from build123d import *

# Parameters (mm, degrees)
F0_W      = 400
F0_H      = 400
F1_DEPTH  = 100
F1_TAPER  = 15
F2_W      = 146.4101615138
F2_H      = 146.4101615138
F3_DEPTH  = 100
F3_TAPER  = 10
F4_R      = 20
F5_R      = 20
F6_DEPTH  = 50
F7_W      = 100
F7_H      = 200
F7_R      = 20
F8_DEPTH  = 10
F9_W      = 100
F9_H      = 10
F10_DEPTH = 75
F11_R     = 5


with BuildPart() as f1:
    # F0 (on Top) → F1 (new body)
    with BuildSketch(Plane.XY):
        with Locations((200, 200)):
            Rectangle(F0_W, F0_H)
    extrude(amount=F1_DEPTH, taper=F1_TAPER)

    # F2 (on face) → F3 (join)
    with BuildSketch(Plane.XY.offset(100)):
        with Locations((200, 200)):
            Rectangle(F2_W, F2_H)
    extrude(amount=F3_DEPTH, taper=F3_TAPER)

    # F4
    f4_edges = [f1.edges().sort_by_distance(p)[0] for p in [
        (13.39746, 13.39746, 50),
        (386.60254, 13.39746, 50),
        (13.39746, 386.60254, 50),
        (386.60254, 386.60254, 50),
        (200, 373.205081, 100),
        (26.794919, 200, 100),
        (200, 26.794919, 100),
        (373.205081, 200, 100),
        (273.205081, 200, 100),
        (200, 126.794919, 100),
        (264.388732, 135.611268, 150),
        (126.794919, 200, 100),
        (135.611268, 135.611268, 150),
        (200, 273.205081, 100),
        (264.388731, 264.388731, 150.000003),
        (135.611268, 264.388732, 150),
    ]]
    fillet(f4_edges, radius=F4_R)

    # F5 (on face) → F6 (join)
    with BuildSketch(Plane.XY.offset(200)):
        with Locations((200, 200)):
            Circle(F5_R)
    extrude(amount=F6_DEPTH)

    # F7 (on face) → F8 (join)
    with BuildSketch(Plane.XY.offset(250)):
        with Locations((200, 200)):
            Rectangle(F7_W, F7_H)
        with Locations((200, 200)):
            Circle(F7_R, mode=Mode.SUBTRACT)
        with Locations((200, 200)):
            Circle(F7_R)
    extrude(amount=F8_DEPTH)

    # F9 (on face) → F10 (join)
    with BuildSketch(Plane.XY.offset(260)):
        with Locations((200, 295)):
            Rectangle(F9_W, F9_H)
    extrude(amount=F10_DEPTH)

    # F11
    f11_edges = [f1.edges().sort_by_distance(p)[0] for p in [
        (200, 290, 260),
        (200, 300, 250),
    ]]
    fillet(f11_edges, radius=F11_R)


solid = f1.part
Read the model definition and answer for the solid it produces. Units are mm, in the model's axes. A direction names the side the tool comes from. Coordinates: 2 decimals unless noted, no trailing zeros. Loops run counter-clockwise (first coordinate to the right, second up) from the corner with the lowest first, then second, coordinate; pieces in that order, holes last.
Q1. The part is cut by section C-C on y = 93. Write down the section's boundary in (x, z), and give its area (3 significant figures).
Q2. Which of the six approach directions +Z, -Z, +X, -X, +Y, -Y give full straight-line access (tool end or side, diameter ignored) to faces 1 (the face through (250, 222, 258)), 2 (the face through (199.292, 263.035, 157.679)), 3 (the face through (150, 222, 258))?
Q3. Consider probe 1 along Z at (x, y) = (267, 322.5); probe 2 along Y at (x, z) = (179, 294.5); probe 3 along Y at (x, z) = (202, 156.5). Determine where each line is inside the solid, lowest interval first.
Q4. The part is cut by section B-B on y = 200. Write down the section's boundary in (x, z), and give its area (3 significant figures).
Q5. Each of these flat-tipped pins is pushed along its axis until it touches: pin 1 Ø5 at (x, z) = (184, 256.5) entering from -Y; pin 2 Ø1 at (x, y) = (278.5, 242) entering from +Z; pin 3 Ø5 at (x, z) = (223.5, 142.5) entering from -Y; pin 4 Ø10 at (x, y) = (146.5, 297) entering from +Z. Where does it stop, or does it pass through?
Q6. The part is cut by section A-A on x = 200. Write down the section's boundary in (y, z), and give its area (3 significant figures).
Q7. The mould has two halves that part along Z. Classify faces 4 (the face through (257.274, 256.969, 158.693)), 5 (the face through (197.79, 370.179, 95.755)), 6 (the face through (199, 290, 300)): +Z half, -Z half, draft (parallel to the pull), parting line (faces both ways), or undercut.
Results below:
1. outline: (0, 0) - (400, 0) - (377.18, 85.18) arc R20 ccw to (357.86, 100) - (42.14, 100) arc R20 ccw to (22.82, 85.18) - close
1. area: 37,200 mm2
2. face 1: +Z, +X, +Y, -Y
2. face 2: +X, -X, +Y
2. face 3: +Z, -X, +Y, -Y
3. probe 1: z = 0 to 100
3. probe 2: y = 290 to 300
3. probe 3: y = 136.76 to 263.24
4. outline: (0, 0) - (400, 0) - (377.18, 85.18) arc R20 ccw to (357.86, 100) - (289.99, 100) arc R20 cw to (270.29, 116.53) - (255.57, 200) - (220, 200) - (220, 250) - (250, 250) - (250, 260) - (150, 260) - (150, 250) - (180, 250) - (180, 200) - (144.43, 200) - (129.71, 116.53) arc R20 cw to (110.01, 100) - (42.14, 100) arc R20 ccw to (22.82, 85.18) - close
4. area: 53,200 mm2
5. pin 1: stops at y = 100
5. pin 2: stops at z = 103.99
5. pin 3: stops at y = 133.85
5. pin 4: stops at z = 335
6. outline: (0, 0) - (400, 0) - (377.18, 85.18) arc R20 ccw to (357.86, 100) - (289.99, 100) arc R20 cw to (270.29, 116.53) - (255.57, 200) - (220, 200) - (220, 250) - (295, 250) arc R5 ccw to (300, 255) - (300, 335) - (290, 335) - (290, 265) arc R5 cw to (285, 260) - (100, 260) - (100, 250) - (180, 250) - (180, 200) - (144.43, 200) - (129.71, 116.53) arc R20 cw to (110.01, 100) - (42.14, 100) arc R20 ccw to (22.82, 85.18) - close
6. area: 55,000 mm2
7. face 4: undercut
7. face 5: +Z half
7. face 6: draft
